from build123d import *

# Parameters (mm, degrees)
F1_DEPTH = 50.8
F3_D     = 25.4
F5_D     = 25.4


with BuildPart() as f1:
    # F0 (on Front) → F1 (new body)
    with BuildSketch(Plane.XZ):
        Polygon((-73.58104, 0), (66.307701, 0), (67.553416, 65.382518), (-73.58104, 65.382518), align=None)
    extrude(amount=F1_DEPTH)

    # F3 (through all)
    with Locations(Plane.XY.offset(65.382518)):
        with Locations((-39.210644, -30.069295)):
            Hole(F3_D / 2)

    # F5 (through all)
    with Locations(Plane.XY.offset(65.382518)):
        with Locations((33.226751, -24.435168)):
            Hole(F5_D / 2)


solid = f1.part
Geometry check sheet. Reference: the model listing, model coordinates, mm. Round coordinates to 2 decimals unless told otherwise and drop trailing zeros. Write each loop counter-clockwise with the first axis right and the second up, starting at its lowest first coordinate (ties: lowest second). Pieces come first, ordered by that corner, then holes.
Item 1: Section check A-A (y = -14.5). Record the boundary of the cut face in (x, z).
Determined:
outline: (-73.58, 0) - (25.32, 0) - (25.32, 65.38) - (-73.58, 65.38) - close; (41.14, 0) - (66.31, 0) - (67.55, 65.38) - (41.14, 65.38) - close
Item 2: Go/stop test with a flat-tipped pin: pin 1 Ø23 at (x, y) = (-39.21, -30.07) entering from -Z. Record where the tip stops, or that it passes through.
Determined:
pin 1: passes through
Item 3: Section check D-D (z = 4.5). Record the boundary of the cut face in (x, y).
Determined:
outline: (-73.58, -50.8) - (66.39, -50.8) - (66.39, 0) - (-73.58, 0) - close; hole circle Ø25.4 at (-39.21, -30.07); hole circle Ø25.4 at (33.23, -24.44)
Item 4: Material ranges on line 1 along Y through (x, z) = (-40, 4); line 2 along X through (y, z) = (-18.5, 35.5); line 3 along X through (y, z) = (-27.5, 33), recorded low to high.
Determined:
line 1: y = -50.8 to -42.74, -17.39 to 0
line 2: x = -73.58 to -44.45, -33.97 to 22, 44.45 to 66.98
line 3: x = -73.58 to -51.65, -26.77 to 20.9, 45.55 to 66.94
Item 5: Section check B-B (x = -46). Record the boundary of the cut face in (y, z).
Determined:
outline: (-50.8, 0) - (-40.8, 0) - (-40.8, 65.38) - (-50.8, 65.38) - close; (-19.34, 0) - (0, 0) - (0, 65.38) - (-19.34, 65.38) - close
Item 6: Section check C-C (z = 58). Record the boundary of the cut face in (x, y), plus the area to 3 significant figures.
Determined:
outline: (-73.58, -50.8) - (67.41, -50.8) - (67.41, 0) - (-73.58, 0) - close; hole circle Ø25.4 at (-39.21, -30.07); hole circle Ø25.4 at (33.23, -24.44)
area: 6,150 mm2
Item 7: Mould release check, pull along X, two halves, no side actions. Record for faces 1 (the face through (-4, -50.8, 33)), 2 (the face through (-51.324, -26.255, 32.234)), 3 (the face through (-73.581, -25, 33)): +X half, -X half, draft (parallel to the pull), parting line (faces both ways), or undercut.
Determined:
face 1: draft
face 2: undercut
face 3: -X half
